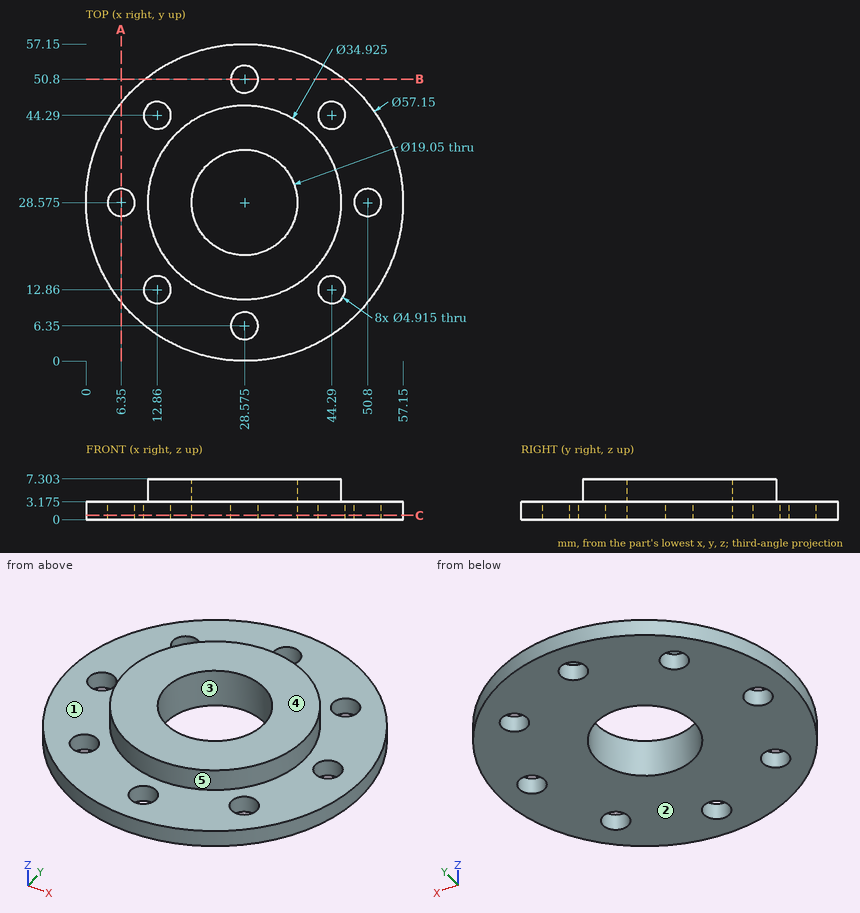
Could you check a few things on this drawing? It's one solid part, dimensions in mm from its lowest x, y, z. A direction names the side the tool comes from. Coordinates: 2 decimals unless noted, no trailing zeros. Order: outer loops, then holes, each group sorted by start corner. A loop starts at its lowest first (then second) coordinate and runs counter-clockwise, first axis right, second up. Notation, with made-up numbers: M -1.5,40 L 57.5,40 A26 cw 57.5,64 Z; hole C 56,38 d5. An arc over 180 degrees is marked long. Use one line per item in the form item = value. Start each with the question number.
1. We'd pull the mould along Y, two halves only. Please class the marked faces 3, 4 and 5: +Y half, -Y half, draft (parallel to the pull), parting line (faces both ways), or undercut.
2. Suppose I cut it at A-A on x = 6.35. Write out the boundary of the cut face in (y, z) (1 decimal).
3. Please list where these lines run through material, in increasing order: line 1 (X direction, y = 29.5, z = 2.25) (1 decimal); line 2 (Y direction, x = 6.35, z = 0.85) (1 decimal); line 3 (Y direction, x = 14, z = 1.5) (1 decimal).
4. Suppose I cut it at C-C on z = 0.75. Count the separate pieces of the cut face and the enclosed holes in it, then the cut area to 3 significant figures.
5. For pin 1 (8 mm diameter, centred on x = 44.29, y = 12.86, fed in from +Z) (1 decimal); pin 2 (2 mm diameter, centred on y = 17, z = 3, fed in from -X), each with a flat end and sliding along its axis, tell me the tip position at first contact or that it passes through.
6. On a 3-axis mill with a long thin cutter (end or side, diameter ignored), from which of +Z, -Z, +X, -X, +Y, -Y can I reach the whole of each face in a straight line? I mean the marked faces 1 and 2. Say none if no direction works.
Geometry says:
q1.face_3 = undercut
q1.face_4 = draft
q1.face_5 = parting line
q2.outline = M 10.6,0 L 26.1,0 L 26.1,3.2 L 10.6,3.2 Z; M 31,0 L 46.5,0 L 46.5,3.2 L 31,3.2 Z
q3.line_1 = 0 to 4.1, 8.6 to 19.1, 38.1 to 48.5, 53.1 to 57.1
q3.line_2 = 10.6 to 26.1, 31 to 46.5
q3.line_3 = 4 to 10.7, 15 to 42.1, 46.5 to 53.2
q4.separate_pieces = 1
q4.enclosed_holes = 9
q4.area = 2,130 mm^2
q5.pin_1 = 3.2
q5.pin_2 = 2.03
q6.face_1 = +Z
q6.face_2 = -Z, +X, -X, +Y, -Y
